Design review of the part built by this model. Coordinates are the model's own, in mm. A direction names the side the tool comes from. Give positions to 0.01 mm unless a question says otherwise; leave off trailing zeros. Loops run counter-clockwise (first coordinate to the right, second up) from the corner with the lowest first, then second, coordinate; pieces in that order, holes last. Notation, with made-up numbers: (-14.5, 74) -> (16.5, 74) arc R19 cw to (16.5, 95) -> close; hole circle Ø10 at (-29, 29). An arc over 180 degrees is marked (long way). Answer as CSV lines item,"result".
from build123d import *

# Parameters (mm, degrees)
F2_R      = 2
F3_W      = 25
F3_H      = 5
F4_DEPTH  = 7.5
F6_DEPTH  = 12.5
F7_R      = 0.2
F9_DEPTH  = 12.5
F10_R     = 1
F11_DEPTH = 5.001


with BuildPart() as f1:
    # F0 (on Right) → F1 (revolve)
    with BuildSketch(Plane.YZ):
        Polygon((-6, 0), (-3.31, 0), (-3.31, 5), (-3.26, 10), (-6, 10), align=None)
    revolve(axis=Axis((0, 0, 28.409811), (0, 0, 1)))

    # F2
    f2_edges = [f1.edges().sort_by_distance(p)[0] for p in [
        (0, 6, 10),
    ]]
    fillet(f2_edges, radius=F2_R)

    # F3 (on Right) → F4 (join, symmetric)
    with BuildSketch(Plane.YZ):
        with Locations((0, -2.5)):
            Rectangle(F3_W, F3_H)
    extrude(amount=F4_DEPTH, both=True)

    # F5 (on Right) → F6 (cut, symmetric)
    with BuildSketch(Plane.YZ):
        with BuildLine():
            Line((-8.5, 0), (-10.5, 0))
            Line((-10.5, 0), (-10.5, -1.5))
            ThreePointArc((-10.5, -1.5), (-10.207107, -2.207107), (-9.5, -2.5))
            Line((-9.5, -2.5), (-7.5, -2.5))
            ThreePointArc((-7.5, -2.5), (-6.519419, -1.696116), (-7.115385, -0.576923))
            Line((-7.115385, -0.576923), (-8.5, 0))
        make_face()
        with BuildLine():
            Line((10.5, 0), (8.5, 0))
            Line((8.5, 0), (7.115385, -0.576923))
            ThreePointArc((7.115385, -0.576923), (6.519419, -1.696116), (7.5, -2.5))
            Line((7.5, -2.5), (9.5, -2.5))
            ThreePointArc((9.5, -2.5), (10.207107, -2.207107), (10.5, -1.5))
            Line((10.5, -1.5), (10.5, 0))
        make_face()
    extrude(amount=F6_DEPTH, both=True, mode=Mode.SUBTRACT)

    # F7
    f7_edges = [f1.edges().sort_by_distance(p)[0] for p in [
        (0, -8.5, 0),
        (0, 8.5, 0),
        (0, -12.5, 0),
        (0, 12.5, 0),
        (0, -12.5, -5),
        (0, 12.5, -5),
    ]]
    fillet(f7_edges, radius=F7_R)

    # F8 (on Right) → F9 (cut, symmetric)
    with BuildSketch(Plane.YZ):
        with BuildLine():
            Line((-4, -5), (4, -5))
            ThreePointArc((4, -5), (0, -3), (-4, -5))
        make_face()
    extrude(amount=F9_DEPTH, both=True, mode=Mode.SUBTRACT)

    # F10 (on face) → F11 (cut, through all)
    with BuildSketch(Plane.XY):
        Circle(F10_R)
    extrude(amount=-F11_DEPTH, mode=Mode.SUBTRACT)


solid = f1.part
Q1. To check wall thickness, follow probe 1 along Y at (x, z) = (-3.75, -2.25); probe 2 along Y at (x, z) = (0, -1.85); probe 3 along X at (y, z) = (0, -1.1). State the ranges of each line that lie inside material, in increasing order. Write a range as from..to.
Filled sheet:
probe 1,"y = -12.5..-10.16, -6.84..6.84, 10.16..12.5"
probe 2,"y = -12.5..-10.44, -6.56..-1, 1..6.56, 10.44..12.5"
probe 3,"x = -7.5..-1, 1..7.5"
Q2. The part is to be moulded in two halves that separate along Y. For faces 1 (the flat face through (7.5, 0, -2)), 2 (the cylindrical face through (2, 0, -3)), 3 (the flat face through (0, -12.5, -3)), say which applies: pulls with the +Y half, pulls with the -Y half, needs draft (parallel to the pull), parting line crosses it, or undercut.
Filled sheet:
face 1,"needs draft"
face 2,"undercut"
face 3,"pulls with the -Y half"
Q3. We need section C-C, the plane z = 0.75. State the section outline as (x, y) points.
Filled sheet:
outline,"circle Ø12 at (0, 0); hole circle Ø6.62 at (0, 0)"
Q4. For faces 4 (the flat face through (0, -11, 0)), 5 (the flat face through (0, 11, 0)), 6 (the cylindrical face through (0.105, 10.199, -2.215)), 7 (the flat face through (5.1, -3.44, 0)), list the 3-axis set-ups (+Z, -Z, +X, -X, +Y, -Y) from which the entire face can be reached by the end or side of a thin tool; tool diameter is ignored.
Filled sheet:
face 4,"+Z, +X, -X, -Y"
face 5,"+Z, +X, -X, +Y"
face 6,"+Z, +X, -X"
face 7,"+Z"
Q5. We need section A-A, the plane z = 7. State the section outline as (x, y) points.
Filled sheet:
outline,"circle Ø12 at (0, 0); hole circle Ø6.58 at (0, 0)"
Q6. Clearance check with flat-ended pins moving along their axes: pin 1 Ø4 at (x, y) = (0, 0) entering from +Z; pin 2 Ø1 at (x, y) = (2, 8.5) entering from +Z; pin 3 Ø5 at (x, z) = (4.5, 8.5) entering from +Y; pin 4 Ø2 at (x, y) = (4.5, 1.5) entering from +Z. State where each tip first meets the part, or that it passes through.
Filled sheet:
pin 1,"stops at z = 0"
pin 2,"stops at z = -2.5"
pin 3,"stops at y = 5.64"
pin 4,"stops at z = 10"
Q7. We need section B-B, the plane y = 9. State the section outline as (x, z) points.
Filled sheet:
outline,"(-7.5, -5) -> (7.5, -5) -> (7.5, -2.5) -> (-7.5, -2.5) -> close"
